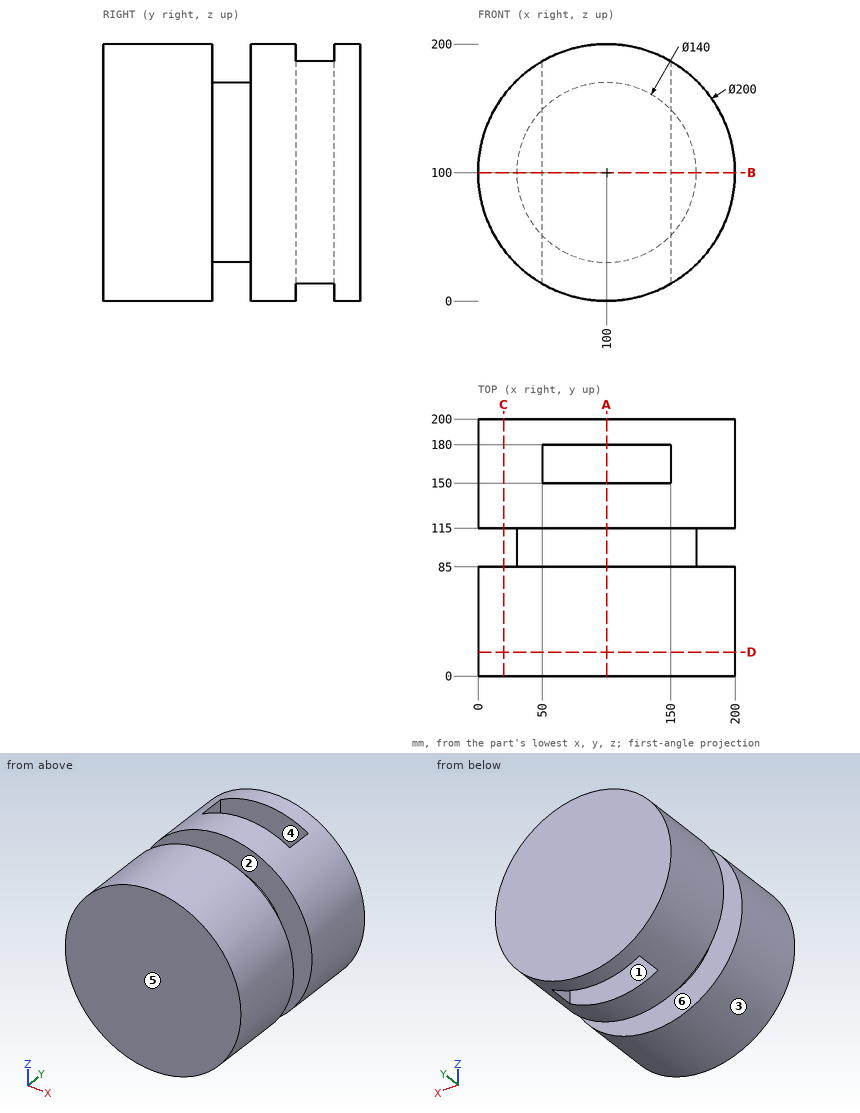
Design review of the part shown in the three views and the two pictorial views. Dimensions are in mm from the part's minimum x, y and z. A direction names the side the tool comes from. Round coordinates to 2 decimals unless told otherwise and drop trailing zeros. Order: outer loops, then holes, each group sorted by start corner. A loop starts at its lowest first (then second) coordinate and runs counter-clockwise, first axis right, second up.
Item 1: Add section A-A, the plane x = 100. State the section outline as (y, z) points.
Working result:
outline: (0, 0) - (85, 0) - (85, 30) - (115, 30) - (115, 0) - (150, 0) - (150, 200) - (115, 200) - (115, 170) - (85, 170) - (85, 200) - (0, 200) - close; (180, 0) - (200, 0) - (200, 200) - (180, 200) - close
Item 2: For pin 1 (2 mm diameter, centred on x = 165, y = 148.5, fed in from -Z); pin 2 (8 mm diameter, centred on x = 114.5, y = 83, fed in from -Z); pin 3 (12 mm diameter, centred on y = 119.5, z = 49.5, fed in from +X); pin 4 (1 mm diameter, centred on x = 107.5, z = 22, fed in from -Y), all flat-tipped, find the tip position at first contact; note any pin that passes through.
Working result:
pin 1: stops at z = 23.16
pin 2: stops at z = 0.55
pin 3: stops at x = 189.55
pin 4: stops at y = 0
Item 3: Machinability: for the marked faces 4, 5 and 6, which of the approach directions +Z, -Z, +X, -X, +Y, -Y give a long, thin tool a straight path to every point of the face, cutting with its end or side? Answer none if there is none.
Working result:
face 4: +Z, -Z
face 5: +Z, -Z, +X, -X, -Y
face 6: none
Item 4: Add section B-B, the plane z = 100. State the section outline as (x, y) points.
Working result:
outline: (0, 0) - (200, 0) - (200, 85) - (170, 85) - (170, 115) - (200, 115) - (200, 200) - (0, 200) - (0, 115) - (30, 115) - (30, 85) - (0, 85) - close; hole (50, 150) - (150, 150) - (150, 180) - (50, 180) - close
Item 5: Add section C-C, the plane x = 20. State the section outline as (y, z) points, and give its area (3 significant figures).
Working result:
outline: (0, 40) - (85, 40) - (85, 160) - (0, 160) - close; (115, 40) - (200, 40) - (200, 160) - (115, 160) - close
area: 20,400 mm2
Item 6: To check wall thickness, follow probe 1 along Y at (x, z) = (148, 117); probe 2 along Y at (x, z) = (127, 31); probe 3 along X at (y, z) = (19, 103). State the ranges of each line that lie inside material, in increasing order.
Working result:
probe 1: y = 0 to 150, 180 to 200
probe 2: y = 0 to 85, 115 to 150, 180 to 200
probe 3: x = 0.05 to 199.95
Item 7: Add section D-D, the plane y = 18.5. State the section outline as (x, z) points, and give its area (3 significant figures).
Working result:
outline: circle Ø200 at (100, 100)
area: 31,400 mm2
Item 8: Draft analysis for pull direction X (two halves, no side actions). For the marked faces 1, 2 and 3, state which applies: released by +X, released by -X, zero draft, split by the parting line, or undercut.
Working result:
face 1: undercut
face 2: zero draft
face 3: split by the parting line
